Here's how the part is built. I have some questions about the finished solid (model axes, mm). Face numbers are marked on the shaded views. Coordinates: 2 decimals unless noted, no trailing zeros. Write each loop counter-clockwise with the first axis right and the second up, starting at its lowest first coordinate (ties: lowest second). Pieces come first, ordered by that corner, then holes. Notation, with made-up numbers: M 84,43.25 L 88,43.25 A24 cw 88,55.25 Z; hole C 38,71 d4. An arc over 180 degrees is marked long. Use one line per item in the form item = value. Start each with the question number.
1. I want a section at B-B, the plane y = -1.25. List the corners of the cut face in (x, z) for me.
2. Please list where these lines run through material, in increasing order: line 1 along X through (y, z) = (-4, 5); line 2 along X through (y, z) = (3, 6.75); line 3 along X through (y, z) = (5.25, 5). Write a range as [from, to].
3. I want a section at D-D, the plane y = -3. List the corners of the cut face in (x, z) for me.
4. Thinking about a two-plate mould opening in X: for the marked faces 1, 2 and 3, which applies, released by +X, released by -X, zero draft, split by the parting line, or undercut?
5. I want a section at C-C, the plane z = 5. List the corners of the cut face in (x, y) for me.
6. I want a section at A-A, the plane x = 15. List the corners of the cut face in (y, z) for me, plus the area to 3 significant figures.
from build123d import *

# Parameters (mm, degrees)
SKETCH1_W           = 40
SKETCH1_H           = 16
BOSS_EXTRUDE1_DEPTH = 10
FILLET1_R           = 2
SKETCH3_R           = 10.05
CUT_EXTRUDE1_DEPTH  = 24.748684174
SKETCH4_R           = 2.55
CUT_EXTRUDE2_DEPTH  = 28.49545417


with BuildPart() as part:
    # Sketch1 → Boss-Extrude1 (new body)
    with BuildSketch(Plane.XY):
        Rectangle(SKETCH1_W, SKETCH1_H)
    extrude(amount=BOSS_EXTRUDE1_DEPTH)

    # Fillet1
    fillet1_edges = [part.edges().sort_by_distance(p)[0] for p in [
        (20, 0, 10),
        (-20, 0, 10),
        (20, 0, 0),
        (-20, 0, 0),
    ]]
    fillet(fillet1_edges, radius=FILLET1_R)

    # Sketch3 → Cut-Extrude1 (cut, through all)
    with BuildSketch(Plane.XY.offset(10)):
        with Locations((0, 8.02)):
            Circle(SKETCH3_R)
    extrude(amount=-CUT_EXTRUDE1_DEPTH, mode=Mode.SUBTRACT)

    # Sketch4 → Cut-Extrude2 (cut, through all)
    with BuildSketch(Plane(origin=(0, 8, 0), x_dir=(1, 0, 0), z_dir=(0, 1, 0))):
        with Locations(Location((-15, -5, 0), (0, 0, 270))):
            Circle(SKETCH4_R)
        with Locations(Location((15, -5, 0), (0, 0, 270))):
            Circle(SKETCH4_R)
    extrude(amount=-CUT_EXTRUDE2_DEPTH, mode=Mode.SUBTRACT)


solid = part.part
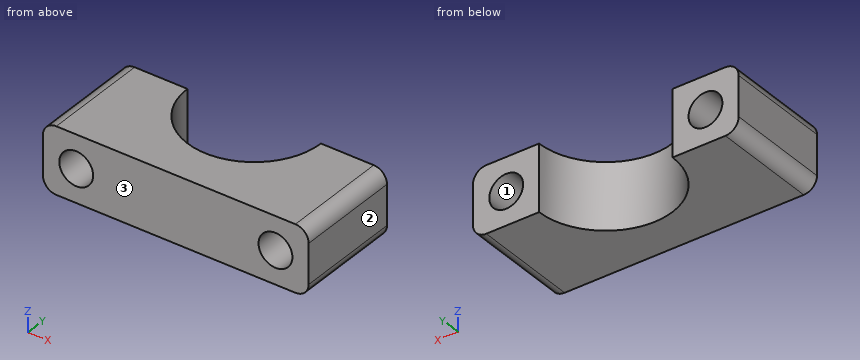
Answer list:
q1.outline = M -20,2 A2 ccw -18,0 L -3.88,0 L -3.88,10 L -18,10 A2 ccw -20,8 Z; M 3.88,0 L 18,0 A2 ccw 20,2 L 20,8 A2 ccw 18,10 L 3.88,10 Z; hole C -15,5 d5.1; hole C 15,5 d5.1
q2.line_1 = [-20, -17.55], [-12.45, 12.45], [17.55, 20]
q2.line_2 = [-20, -16.85], [-13.15, -8.71], [8.71, 13.15], [16.85, 20]
q2.line_3 = [-20, -17.55], [-12.45, -9.66], [9.66, 12.45], [17.55, 20]
q3.outline = M -20,2 A2 ccw -18,0 L 18,0 A2 ccw 20,2 L 20,8 A2 ccw 18,10 L -18,10 A2 ccw -20,8 Z; hole C -15,5 d5.1; hole C 15,5 d5.1
q4.face_1 = undercut
q4.face_2 = released by +X
q4.face_3 = zero draft
q5.outline = M -20,-8 L -17.55,-8 L -17.55,8 L -20,8 Z; M -12.45,-8 L 12.45,-8 L 12.45,8 L 10.05,8 A10.05 cw -10.05,8 L -12.45,8 Z; M 17.55,-8 L 20,-8 L 20,8 L 17.55,8 Z
q6.outline = M -8,0 L 8,0 L 8,2.45 L -8,2.45 Z; M -8,7.55 L 8,7.55 L 8,10 L -8,10 Z
q6.area = 78.4 mm²
